The model under review builds one solid part; all positions refer to its coordinate system, in mm. A direction names the side the tool comes from. Round coordinates to 2 decimals unless told otherwise and drop trailing zeros. Order: outer loops, then holes, each group sorted by start corner. A loop starts at its lowest first (then second) coordinate and runs counter-clockwise, first axis right, second up. Notation, with made-up numbers: (81, -13.5) -> (105, -13.5) arc R10 ccw to (105, -5.5) -> close; hole circle Ø1 at (1.5, -38). An arc over 180 degrees is marked (long way). Return JSON: item names as keys, results as strings. Group by question number.
from build123d import *

# Parameters (mm, degrees)
F0_W           = 215
F0_H           = 114
F1_DEPTH       = 50
F2_T           = -2
F3_W           = 20
F3_H           = 110
F3_R           = 30
F4_DEPTH       = 2
F8_D           = 3.2
F8_DEPTH       = 2
F8_TIP         = 0.9613769904
F8_ON_F5_D     = 3.2
F8_ON_F5_DEPTH = 2
F8_ON_F5_TIP   = 0.9613769904
F8_ON_F6_D     = 3.2
F8_ON_F6_DEPTH = 2
F8_ON_F6_TIP   = 0.9613769904


with BuildPart() as f1:
    # F0 (on Top) → F1 (new body)
    with BuildSketch(Plane.XY):
        Rectangle(F0_W, F0_H)
    extrude(amount=F1_DEPTH)

    # F2
    f2_openings = [f1.faces().sort_by_distance(p)[0] for p in [
        (-107.5, 0, 25),
    ]]
    offset(amount=F2_T, openings=f2_openings)

    # F3 (on face) → F4 (cut, through all)
    with BuildSketch(Plane.XY.offset(50)):
        with Locations((-97.5, 0)):
            Rectangle(F3_W, F3_H)
        with Locations((59.5, 20)):
            Circle(F3_R)
    extrude(amount=-F4_DEPTH, mode=Mode.SUBTRACT)

    # F8
    with Locations(Plane(origin=(0, 0, 0), x_dir=(1, 0, 0), z_dir=(0, 0, -1))):
        with Locations((-74.5, 25), (-74.5, -25), (75.5, -25), (75.5, 25)):
            Hole(F8_D / 2, depth=F8_DEPTH)
            with Locations((0, 0, -(F8_DEPTH + F8_TIP / 2))):  # 118° drill point
                Cone(0, F8_D / 2, F8_TIP, mode=Mode.SUBTRACT)

    # F8 on F5
    with Locations(Plane.XZ.offset(57)):
        with Locations((-71.1912775098, 37), (-71.1912775098, 12), (67.8294761911, 37), (67.8294761911, 12)):
            Hole(F8_ON_F5_D / 2, depth=F8_ON_F5_DEPTH)
            with Locations((0, 0, -(F8_ON_F5_DEPTH + F8_ON_F5_TIP / 2))):  # 118° drill point
                Cone(0, F8_ON_F5_D / 2, F8_ON_F5_TIP, mode=Mode.SUBTRACT)

    # F8 on F6
    with Locations(Plane(origin=(0, 57, 0), x_dir=(-1, 0, 0), z_dir=(0, 1, 0))):
        with Locations((71.1912775098, 12), (-67.8294761911, 12)):
            Hole(F8_ON_F6_D / 2, depth=F8_ON_F6_DEPTH)
            with Locations((0, 0, -(F8_ON_F6_DEPTH + F8_ON_F6_TIP / 2))):  # 118° drill point
                Cone(0, F8_ON_F6_D / 2, F8_ON_F6_TIP, mode=Mode.SUBTRACT)


solid = f1.part
Item 1: Consider section B-B on x = -91. State the section outline as (y, z) points.
Item 2: Wall thickness on line 1 along X through (y, z) = (55.5, 12); line 2 along X through (y, z) = (-25, 1.3); line 3 along Y through (x, z) = (-74.5, 1.05): over which ranges is each line inside the solid? List them lowest first.
Item 3: For faces 1 (the face through (55.595, 49.745, 49.014)), 2 (the face through (-2, 1, 2)), 3 (the face through (-107.5, -26, 1)), list the 3-axis set-ups (+Z, -Z, +X, -X, +Y, -Y) from which the entire face can be reached by the end or side of a thin tool; tool diameter is ignored.
Item 4: Consider section C-C on z = 21. State the section outline as (x, y) points.
Item 5: Consider section D-D on x = -58. State the section outline as (y, z) points, plus the area to 3 significant figures.
Item 6: Consider section A-A on y = 20. State the section outline as (x, z) points, plus the area to 3 significant figures.
Item 7: Insertion check: pin 1 Ø1.9 at (x, z) = (67.83, 37) entering from -Y; pin 2 Ø14 at (y, z) = (-24.5, 23.5) entering from -X; pin 3 Ø3 at (x, y) = (-74.5, -25) entering from -Z. Each pin has a flat end and moves straight along its axis. Give the tip position at first contact, or say it passes through.
Item 8: The part is to be moulded in two halves that separate along Z. For faces 4 (the face through (-2, 1, 0)), 5 (the face through (107.5, -1, 25)), 6 (the face through (-2, -55, 26)), say which applies: +Z half, -Z half, draft (parallel to the pull), parting line (faces both ways), or undercut.
Values:
{
 "1": {"outline": "(-57, 0) -> (57, 0) -> (57, 50) -> (55, 50) -> (55, 2) -> (-55, 2) -> (-55, 50) -> (-57, 50) -> close"},
 "2": {"line 1": "-107.5 to -72.79, -69.59 to 66.23, 69.43 to 107.5", "line 2": "-107.5 to -76.1, -72.9 to 73.9, 77.1 to 107.5", "line 3": "-57 to -26.6, -23.4 to 23.4, 26.6 to 57"},
 "3": {"face 1": "+Z", "face 2": "-X", "face 3": "+Z, -Z, -X, +Y, -Y"},
 "4": {"outline": "(-107.5, -57) -> (107.5, -57) -> (107.5, 57) -> (-107.5, 57) -> (-107.5, 55) -> (105.5, 55) -> (105.5, -55) -> (-107.5, -55) -> close"},
 "5": {"outline": "(-57, 0) -> (57, 0) -> (57, 50) -> (-57, 50) -> close; hole (-55, 2) -> (55, 2) -> (55, 48) -> (-55, 48) -> close", "area": "640 mm^2"},
 "6": {"outline": "(-107.5, 0) -> (107.5, 0) -> (107.5, 50) -> (89.5, 50) -> (89.5, 48) -> (105.5, 48) -> (105.5, 2) -> (-107.5, 2) -> close; (-87.5, 48) -> (29.5, 48) -> (29.5, 50) -> (-87.5, 50) -> close", "area": "792 mm^2"},
 "7": {"pin 1": "y = 55", "pin 2": "x = 105.5", "pin 3": "z = 48"},
 "8": {"face 4": "-Z half", "face 5": "draft", "face 6": "undercut"}
}
